Build history of the part. All positions in model axes, mm. Give positions to 0.01 mm unless a question says otherwise; leave off trailing zeros. Put each result on its own line as item: value.
from build123d import *

# Parameters (mm, degrees)
F1_DEPTH = 330
F2_R     = 1
F3_R     = 0.5
F4_R     = 0.1


with BuildPart() as f1:
    # F0 (on Top) → F1 (new body)
    with BuildSketch(Plane.XY):
        with BuildLine():
            Line((-0.025, 4.0583112277), (-2.2905442747, 4.0583112277))
            Line((-2.2905442747, 4.0583112277), (-5.8640526549, 7.6318196079))
            Line((-5.8640526549, 7.6318196079), (-3, 7.6318196079))
            Line((-3, 7.6318196079), (-3, 10))
            Line((-3, 10), (-10, 10))
            Line((-10, 10), (-10, 3))
            Line((-10, 3), (-7.6318196079, 3))
            Line((-7.6318196079, 3), (-7.6318196079, 5.8640526549))
            Line((-7.6318196079, 5.8640526549), (-4, 2.232233047))
            Line((-4, 2.232233047), (-4, 0.025))
            Line((-4, 0.025), (-2.8230957687, 0.025))
            Line((-2.8230957687, 0.025), (-2.8230957687, 0.7926485917))
            Line((-2.8230957687, 0.7926485917), (-1.8740334308, 1.411684829))
            ThreePointArc((-1.8740334308, 1.411684829), (-2.3460869309, 0.0270456781), (-1.906078865, -1.3681077138))
            Line((-1.906078865, -1.3681077138), (-2.8238623803, -0.7794121329))
            Line((-2.8238623803, -0.7794121329), (-2.8238623803, -0.025))
            Line((-2.8238623803, -0.025), (-4, -0.025))
            Line((-4, -0.025), (-4, -2.232233047))
            Line((-4, -2.232233047), (-7.6318196079, -5.8640526549))
            Line((-7.6318196079, -5.8640526549), (-7.6318196079, -3))
            Line((-7.6318196079, -3), (-10, -3))
            Line((-10, -3), (-10, -10))
            Line((-10, -10), (-3, -10))
            Line((-3, -10), (-3, -7.6318196079))
            Line((-3, -7.6318196079), (-5.8640526549, -7.6318196079))
            Line((-5.8640526549, -7.6318196079), (-2.232233047, -4))
            Line((-2.232233047, -4), (-0.05, -4))
            Line((-0.05, -4), (-0.05, -2.9588690959))
            Line((-0.05, -2.9588690959), (-0.7483266194, -2.9588690959))
            Line((-0.7483266194, -2.9588690959), (-1.5537911294, -1.7580069631))
            ThreePointArc((-1.5537911294, -1.7580069631), (-0.0257632285, -2.3461013645), (1.5148107083, -1.7917041816))
            Line((1.5148107083, -1.7917041816), (0.7406048023, -2.9588690959))
            Line((0.7406048023, -2.9588690959), (0.05, -2.9588690959))
            Line((0.05, -2.9588690959), (0.05, -4))
            Line((0.05, -4), (2.232233047, -4))
            Line((2.232233047, -4), (5.8640526549, -7.6318196079))
            Line((5.8640526549, -7.6318196079), (3, -7.6318196079))
            Line((3, -7.6318196079), (3, -10))
            Line((3, -10), (10, -10))
            Line((10, -10), (10, -3))
            Line((10, -3), (7.6318196079, -3))
            Line((7.6318196079, -3), (7.6318196079, -5.8640526549))
            Line((7.6318196079, -5.8640526549), (4, -2.232233047))
            Line((4, -2.232233047), (4, -0.025))
            Line((4, -0.025), (2.8238623803, -0.025))
            Line((2.8238623803, -0.025), (2.8238623803, -0.7921485609))
            Line((2.8238623803, -0.7921485609), (1.8740334308, -1.411684829))
            ThreePointArc((1.8740334308, -1.411684829), (2.3460040432, 0.0334721598), (1.8329957125, 1.4645757318))
            Line((1.8329957125, 1.4645757318), (2.8230957687, 0.8068363719))
            Line((2.8230957687, 0.8068363719), (2.8230957687, 0.025))
            Line((2.8230957687, 0.025), (4, 0.025))
            Line((4, 0.025), (4, 2.232233047))
            Line((4, 2.232233047), (7.6318196079, 5.8640526549))
            Line((7.6318196079, 5.8640526549), (7.6318196079, 3))
            Line((7.6318196079, 3), (10, 3))
            Line((10, 3), (10, 10))
            Line((10, 10), (3, 10))
            Line((3, 10), (3, 7.6318196079))
            Line((3, 7.6318196079), (5.8640526549, 7.6318196079))
            Line((5.8640526549, 7.6318196079), (2.2905442747, 4.0583112277))
            Line((2.2905442747, 4.0583112277), (0.025, 4.0583112277))
            Line((0.025, 4.0583112277), (0.025, 2.9460287187))
            Line((0.025, 2.9460287187), (0.7554459771, 2.9460287187))
            Line((0.7554459771, 2.9460287187), (1.5118729288, 1.7941838266))
            ThreePointArc((1.5118729288, 1.7941838266), (-0.0195250931, 2.3461615731), (-1.5415243666, 1.7687730164))
            Line((-1.5415243666, 1.7687730164), (-0.7608180556, 2.9474266339))
            Line((-0.7608180556, 2.9474266339), (-0.025, 2.9474266339))
            Line((-0.025, 2.9474266339), (-0.025, 4.0583112277))
        make_face()
    extrude(amount=F1_DEPTH)

    # F2
    f2_edges = [f1.edges().sort_by_distance(p)[0] for p in [
        (10, 10, 165),
        (10, -10, 165),
        (-10, -10, 165),
        (-3, -10, 165),
        (3, -10, 165),
        (-3, 10, 165),
        (-10, 3, 165),
        (10, 3, 165),
        (10, -3, 165),
        (-10, -3, 165),
        (-10, 10, 165),
        (3, 10, 165),
    ]]
    fillet(f2_edges, radius=F2_R)

    # F3
    f3_edges = [f1.edges().sort_by_distance(p)[0] for p in [
        (-7.63182, 5.864053, 165),
        (-5.864053, 7.63182, 165),
        (5.864053, 7.63182, 165),
        (7.63182, 5.864053, 165),
        (-7.63182, -5.864053, 165),
        (-5.864053, -7.63182, 165),
        (5.864053, -7.63182, 165),
        (7.63182, -5.864053, 165),
    ]]
    fillet(f3_edges, radius=F3_R)

    # F4
    f4_edges = [f1.edges().sort_by_distance(p)[0] for p in [
        (-1.874033, 1.411685, 165),
        (2.290544, 4.058311, 165),
        (4.656946, 7.63182, 165),
        (-1.541524, 1.768773, 165),
        (1.514811, -1.791704, 165),
        (1.874033, -1.411685, 165),
        (1.832996, 1.464576, 165),
        (1.511873, 1.794184, 165),
        (-1.906079, -1.368108, 165),
        (-1.553791, -1.758007, 165),
    ]]
    fillet(f4_edges, radius=F4_R)


solid = f1.part
1) Wall check: L1, parallel to X at y = 0.5, z = 295; L2, parallel to Y at x = 0.5, z = 285.5; L3, parallel to X at y = -8.25, z = 301. Give the ranges that are in metal, low to high.
Filled sheet:
L1: -4 to -2.82, -2.29 to 2.29, 2.82 to 4
L2: -4 to -2.96, -2.29 to 2.29, 2.95 to 4.06
L3: -10 to -3, 3 to 10
2) Pin check, flat tips, straight feed: pin 1 (0.8 mm diameter, centred on x = 0.5, z = 221, fed in from +Y); pin 2 (0.6 mm diameter, centred on x = 0.5, z = 117.5, fed in from -Y); pin 3 (0.5 mm diameter, centred on y = -3.5, z = 208.5, fed in from -X). Stop position of each tip, or through.
Filled sheet:
pin 1: y = 4.06
pin 2: y = -4
pin 3: x = -9.97
3) Pull direction Z, two halves, no side cores. Call faces 1 (the flat face through (0, 0, 330)), 2 (the flat face through (0, 0, 0)), 3 (the flat face through (-10, 7, 163)): released by +Z, released by -Z, zero draft, split by the parting line, or undercut.
Filled sheet:
face 1: released by +Z
face 2: released by -Z
face 3: zero draft
